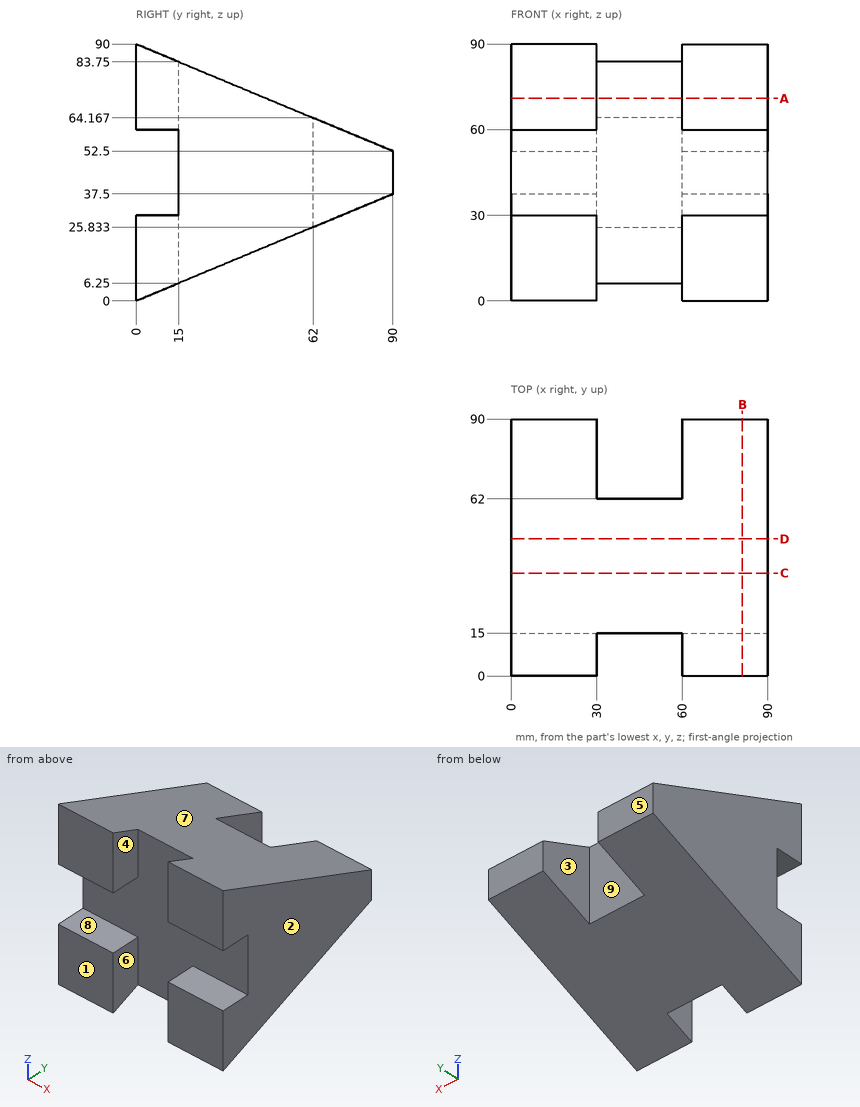
Answer from the drawing. Dimensions are ordinates in mm from the lowest x, y and z of the part. A direction names the side the tool comes from. Coordinates: 2 decimals unless noted, no trailing zeros. Order: outer loops, then holes, each group sorted by start corner. A loop starts at its lowest first (then second) coordinate and runs counter-clockwise, first axis right, second up. Notation, with made-up numbers: (5.25, 20) - (25.25, 20) arc R24 ccw to (25.25, 57) - close; hole circle Ø2 at (15, 67). An arc over 180 degrees is marked (long way). Put each result on its own line as item: value. Start each with the question number.
1) For the marked faces 5, 6, 7, 8 and 9, determine the directions among +Z, -Z, +X, -X, +Y, -Y from which every point of the face is accessible in a straight line to the end or side of a thin tool.
2) Flat-ended cylindrical pins translate along their axes: pin 1 (9 mm diameter, centred on x = 51, z = 44.5, fed in from +Y); pin 2 (7.5 mm diameter, centred on x = 20.5, y = 7, fed in from +Z); pin 3 (7.5 mm diameter, centred on x = 13, y = 4, fed in from -Z). Find the tip coordinate at first contact, or state that the pin passes through.
3) For a pull along X with two mould halves and no side action, classify the marked faces 1, 2, 3 and 4 as released by +X, released by -X, zero draft, split by the parting line, or undercut.
4) Find the intervals of material crossed by line 1 (X direction, y = 63, z = 55); line 2 (Z direction, x = 15.5, y = 9); line 3 (Z direction, x = 63.5, y = 7.5) (1 decimal), in increasing order. Write a range as from..to.
5) Find section D-D (y = 48). Give the vertices of the cut face in (x, z), plus the area to 3 significant figures.
6) Find section B-B (x = 81). Give the vertices of the cut face in (y, z), plus the area to 4 significant figures.
7) Find section A-A (z = 71). Give the vertices of the cut face in (x, y).
8) Find section C-C (y = 36). Give the vertices of the cut face in (x, z).
Results list:
1. face 5: +Z, -Z, +X, -X, +Y
1. face 6: +Z, -Z, -Y
1. face 7: +Z, +X, -X, +Y
1. face 8: +X, -X, -Y
1. face 9: +Z, -Z, +Y
2. pin 1: stops at y = 62
2. pin 2: stops at z = 88.65
2. pin 3: stops at z = 0.1
3. face 1: zero draft
3. face 2: released by +X
3. face 3: undercut
3. face 4: undercut
4. line 1: x = 0..30, 60..90
4. line 2: z = 3.75..30, 60..86.25
4. line 3: z = 3.1..30, 60..86.9
5. outline: (0, 20) - (90, 20) - (90, 70) - (0, 70) - close
5. area: 4,500 mm^2
6. outline: (0, 0) - (90, 37.5) - (90, 52.5) - (0, 90) - (0, 60) - (15, 60) - (15, 30) - (0, 30) - close
6. area: 4,275 mm^2
7. outline: (0, 0) - (30, 0) - (30, 15) - (60, 15) - (60, 0) - (90, 0) - (90, 45.6) - (0, 45.6) - close
8. outline: (0, 15) - (90, 15) - (90, 75) - (0, 75) - close
